```python
from build123d import *

# Parameters (mm, degrees)
SKETCH1_R           = 19.05
SKETCH1_R_2         = 6.35
BOSS_EXTRUDE1_DEPTH = 9.398
SKETCH4_W           = 38.1
SKETCH4_H           = 9.398
BOSS_EXTRUDE3_DEPTH = 44.45
FILLET1_R           = 19.05
FILLET2_R           = 9.398
CUT_EXTRUDE1_REACH  = 122.111
SKETCH6_R           = 6.35


with BuildPart() as part:
    # Sketch1 → Boss-Extrude1 (new body)
    with BuildSketch(Plane(origin=(0, 0, 0), x_dir=(1, 0, 0), z_dir=(0, 1, 0))):
        with BuildLine():
            Line((-23.785306473, 25.4), (-88.9, 25.4))
            Line((-88.9, 25.4), (-88.9, -25.4))
            Line((-88.9, -25.4), (-23.785306473, -25.4))
            ThreePointArc((-23.785306473, -25.4), (34.798, 0), (-23.785306473, 25.4))
        make_face()
        with Locations(Location((0, 0, 0), (0, 0, 270))):
            Circle(SKETCH1_R, mode=Mode.SUBTRACT)
        with Locations(Location((-69.85, 0, 0), (0, 0, 270))):
            Circle(SKETCH1_R_2, mode=Mode.SUBTRACT)
    extrude(amount=BOSS_EXTRUDE1_DEPTH)

    # Sketch4 → Boss-Extrude3 (add)
    with BuildSketch(Plane(origin=(0, 9.398, 0), x_dir=(1, 0, 0), z_dir=(0, 1, 0))):
        with Locations((-69.85, 20.701)):
            Rectangle(SKETCH4_W, SKETCH4_H)
        with Locations((-69.85, -20.701)):
            Rectangle(SKETCH4_W, SKETCH4_H)
    extrude(amount=BOSS_EXTRUDE3_DEPTH)

    # Fillet1
    fillet1_edges = [part.edges().sort_by_distance(p)[0] for p in [
        (-88.9, 53.848, 20.701),
        (-88.9, 53.848, -20.701),
        (-50.8, 53.848, -20.701),
        (-50.8, 53.848, 20.701),
    ]]
    fillet(fillet1_edges, radius=FILLET1_R - 0.0001)  # a hair under: the kernel refuses the full size

    # Fillet2
    fillet2_edges = [part.edges().sort_by_distance(p)[0] for p in [
        (-23.785306473, 4.699, 25.4),
        (-23.785306473, 4.699, -25.4),
        (-50.8, 9.398, -20.701),
        (-50.8, 9.398, 20.701),
    ]]
    fillet(fillet2_edges, radius=FILLET2_R)

    # Cut-Extrude1: up to this face of the body (flat: up to its plane)
    cut_extrude1_end = Plane(part.part.faces().sort_by_distance((-66.468021602, 22.831221423, -25.4))[0])
    # Sketch6 → Cut-Extrude1 (cut, up to the picked face)
    with BuildSketch(Plane.XY.offset(25.4), mode=Mode.PRIVATE) as cut_extrude1_sk1:
        with Locations((-69.85, 34.798)):
            Circle(SKETCH6_R)
    cut_extrude1_tool1 = split(extrude(cut_extrude1_sk1.sketch, amount=-CUT_EXTRUDE1_REACH, mode=Mode.PRIVATE), bisect_by=cut_extrude1_end, keep=Keep.BOTH, mode=Mode.PRIVATE)
    add(cut_extrude1_tool1.solids().sort_by(Axis((-69.85, 34.798, 25.4), (0, 0, -1)))[0], mode=Mode.SUBTRACT)


solid = part.part
```
Geometry check sheet. Reference: the model listing, model coordinates, mm. A direction names the side the tool comes from. Coordinates: 2 decimals unless noted, no trailing zeros. Write each loop counter-clockwise with the first axis right and the second up, starting at its lowest first coordinate (ties: lowest second). Pieces come first, ordered by that corner, then holes. Notation, with made-up numbers: M -5.75,4.25 L 44.25,4.25 A16 cw 44.25,32.25 Z; hole C -6.5,1 d7. An arc over 180 degrees is marked long. One line per item, written item: value. Start each with the question number.
(1) Scan lines: line 1 along X through (y, z) = (3, 0); line 2 along Z through (x, y) = (-77, 33.5); line 3 along Y through (x, z) = (-69.85, 20.5). Record each from-to range of solid material in increasing order. Write a range as [from, to].
(2) Sectioned sample at B-B, the plane y = 7. Enter the section's corners in (x, z).
(3) Sectioned sample at C-C, the plane x = 0. Enter the section's corners in (y, z).
(4) Depth check by flat-ended pin: pin 1 (7.5 mm diameter, centred on y = 28.5, z = -20.5, fed in from +X); pin 2 (10 mm diameter, centred on x = -69.85, z = 0, fed in from +Y); pin 3 (16.5 mm diameter, centred on x = -69.85, y = 34.798, fed in from -Z); pin 4 (14.5 mm diameter, centred on x = -69.85, y = 34.798, fed in from +Z). Enter the tip coordinate at first touch or a pass-through.
(5) Sectioned sample at D-D, the plane z = -12. Enter the section's corners in (x, y), and give its area (3 significant figures).
(6) Tool access check on faces 1 (the face through (-71, 26, 16.002)), 2 (the face through (-50.8, 27, -21)), 3 (the face through (-65, 21, -25.4)), 4 (the face through (-28, 9.398, 0)). Record the directions out of +Z, -Z, +X, -X, +Y, -Y that give a thin tool (end or side, any length) a straight path to the whole face; none if there is none.
(7) Sectioned sample at A-A, the plane z = 0. Enter the section's corners in (x, y), and give its area (3 significant figures).
(8) Release check for a two-part mould opening along Z. For faces 5 (the face through (-11.59, 4.63, -15.12)), 6 (the face through (-56.23, 48.12, -20.77)), 7 (the face through (-24.22, 4.76, 25.9)) record: released by +Z, released by -Z, zero draft, split by the parting line, or undercut.
Filled sheet:
1. line 1: [-88.9, -76.2], [-63.5, -19.05], [19.05, 34.8]
1. line 2: [-25.4, -16], [16, 25.4]
1. line 3: [0, 28.45], [41.15, 53.85]
2. outline: M -88.9,-25.4 L -27.25,-25.4 A9.4 cw -21.45,-27.4 A34.8 ccw long -21.45,27.4 A9.4 cw -27.25,25.4 L -88.9,25.4 Z; hole C -69.85,0 d12.7; hole C 0,0 d38.1
3. outline: M 0,-34.8 L 9.4,-34.8 L 9.4,-19.05 L 0,-19.05 Z; M 0,19.05 L 9.4,19.05 L 9.4,34.8 L 0,34.8 Z
4. pin 1: x = -50.8
4. pin 2: through
4. pin 3: z = -25.4
4. pin 4: z = 25.4
5. outline: M -88.9,0 L -14.8,0 L -14.8,9.4 L -88.9,9.4 Z; M 14.8,0 L 32.66,0 L 32.66,9.4 L 14.8,9.4 Z
5. area: 864 mm²
6. face 1: +X, -X, +Y
6. face 2: +Z, -Z, +X, +Y
6. face 3: -Z, -X, +Y, -Y
6. face 4: +X, +Y
7. outline: M -88.9,0 L -76.2,0 L -76.2,9.4 L -88.9,9.4 Z; M -63.5,0 L -19.05,0 L -19.05,9.4 L -63.5,9.4 Z; M 19.05,0 L 34.8,0 L 34.8,9.4 L 19.05,9.4 Z
7. area: 685 mm²
8. face 5: undercut
8. face 6: zero draft
8. face 7: released by +Z
